Check sheet for the modelled part. Datum: model origin and axes. Units: mm. A direction names the side the tool comes from. Give positions to 0.01 mm unless a question says otherwise; leave off trailing zeros. Order: outer loops, then holes, each group sorted by start corner. A loop starts at its lowest first (then second) coordinate and runs counter-clockwise, first axis right, second up.
Autodesk Inventor part; units mm, degrees
ref_plane "YZ Plane" through (0, 0, 0) normal (1, 0, 0) x (0, 1, 0)
ref_plane "XZ Plane" through (0, 0, 0) normal (0, 1, 0) x (-1, 0, 0)
ref_plane "XY Plane" through (0, 0, 0) normal (0, 0, 1) x (1, 0, 0)
sketch "Sketch2" plane through (0, 0, 0) normal (0, 1, 0) x (-1, 0, 0)
  line L0 (-200, -150) -> (200, -150)
  line L1 (200, -150) -> (200, -200)
  line L2 (-200, -200) -> (-200, -150)
  line L3 (0, -269.3547) -> (0, -73.2831)
  line L4 (200, -200) -> (200, -270)
  line L5 (200, -270) -> (-200, -270)
  line L6 (-200, -270) -> (-200, -200)
  line L7 (200, -150) -> (412.132, 62.132)
  line L8 (200, -150) -> (500, -150) construction
  line L9 (412.132, 62.132) -> (412.132, -57.868)
  line L10 (412.132, -57.868) -> (200, -270)
  line L11 (-200, -150) -> (-412.132, 62.132)
  line L12 (-412.132, 62.132) -> (-412.132, -57.868)
  line L13 (-412.132, -57.868) -> (-200, -270)
  point P0 (0, 0)
  point P1 (0, -175)
  point P2 (412.5, 61.0149)
  dimension "d9" = 400
  dimension "d10" = 50
  dimension "d39" = 70
  dimension "d40" = 200
  dimension "d41" = 45
  dimension "d42" = 120
  dimension "d43" = 150
  dimension "d51" = 300
extrude "Extrusion2" add sketch "Sketch2" along normal blind 150
sketch "Sketch8" plane through (0, 0, 0) normal (0, -1, 0) x (1, 0, 0)
  line L0 (412.132, -57.868) -> (200, -270)
  line L1 (200, -270) -> (-200, -270)
  line L2 (-200, -270) -> (-412.132, -57.868)
  line L3 (-412.132, -57.868) -> (-412.132, 62.132)
  line L4 (-412.132, 62.132) -> (-200, -150)
  line L5 (-200, -150) -> (200, -150)
  line L6 (200, -150) -> (412.132, 62.132)
  line L7 (412.132, 62.132) -> (412.132, -57.868)
  line L8 (-412.132, 62.132) -> (-412.132, 242.132)
  line L9 (412.132, 62.132) -> (412.132, 242.132)
  line L10 (-412.132, 62.132) -> (-412.132, -57.868)
  line L11 (-412.132, -57.868) -> (-200, -270)
  line L12 (-200, -270) -> (200, -270)
  line L13 (200, -270) -> (412.132, -57.868)
  line L14 (412.132, -57.868) -> (412.132, 62.132)
  line L15 (50, 242.132) -> (50, 49.557)
  line L16 (50, 49.557) -> (-50, 49.557)
  line L17 (-50, 49.557) -> (-50, 242.132)
  line L18 (412.132, 242.132) -> (50, 242.132)
  line L19 (-50, 242.132) -> (-412.132, 242.132)
  dimension "d45" = 180
  dimension "d46" = 180
  dimension "d47" = 100
extrude "Extrusion9" add sketch "Sketch8" along normal blind 4
sketch "Sketch9" plane through (0, -4, 0) normal (0, -1, 0) x (1, 0, 0)
  line L0 (200, -270) -> (-200, -270)
  line L1 (-200, -270) -> (-412.132, -57.868)
  line L2 (-412.132, -57.868) -> (-412.132, 242.132)
  line L3 (-412.132, 242.132) -> (-50, 242.132)
  line L4 (-50, 242.132) -> (-50, 49.557)
  line L5 (-50, 49.557) -> (50, 49.557)
  line L6 (50, 49.557) -> (50, 242.132)
  line L7 (50, 242.132) -> (412.132, 242.132)
  line L8 (412.132, 242.132) -> (412.132, -57.868)
  line L9 (412.132, -57.868) -> (200, -270)
  line L10 (200, -270) -> (-200, -270)
  line L11 (-200, -270) -> (-412.132, -57.868)
  line L12 (-412.132, -57.868) -> (-412.132, 242.132)
  line L13 (-412.132, 242.132) -> (-50, 242.132)
  line L14 (-50, 242.132) -> (-50, 49.557)
  line L15 (-50, 49.557) -> (50, 49.557)
  line L16 (50, 49.557) -> (50, 242.132)
  line L17 (50, 242.132) -> (412.132, 242.132)
  line L18 (412.132, 242.132) -> (412.132, -57.868)
  line L19 (412.132, -57.868) -> (200, -270)
  line L20 (200, -270) -> (-200, -270)
  line L21 (-200, -270) -> (-412.132, -57.868)
  line L22 (-412.132, -57.868) -> (-412.132, 242.132)
  line L23 (-412.132, 242.132) -> (-50, 242.132)
  line L24 (-50, 242.132) -> (-50, 49.557)
  line L25 (-50, 49.557) -> (50, 49.557)
  line L26 (50, 49.557) -> (50, 242.132)
  line L27 (50, 242.132) -> (412.132, 242.132)
  line L28 (412.132, 242.132) -> (412.132, -57.868)
  line L29 (412.132, -57.868) -> (200, -270)
  line L30 (250, 110) -> (250, 190)
  line L31 (200, -150) -> (412.132, 62.132)
  line L32 (-200, -150) -> (200, -150)
  line L33 (-412.132, 62.132) -> (-200, -150)
  line L34 (-412.132, 242.132) -> (-412.132, 62.132)
  line L35 (-50, 242.132) -> (-412.132, 242.132)
  line L36 (-50, 49.557) -> (-50, 242.132)
  line L37 (50, 49.557) -> (-50, 49.557)
  line L38 (50, 242.132) -> (50, 49.557)
  line L39 (412.132, 242.132) -> (50, 242.132)
  line L40 (412.132, 62.132) -> (412.132, 242.132)
  line L41 (200, -150) -> (412.132, 62.132)
  line L42 (-200, -150) -> (200, -150)
  line L43 (-412.132, 62.132) -> (-200, -150)
  line L44 (-412.132, 242.132) -> (-412.132, 62.132)
  line L45 (-50, 242.132) -> (-412.132, 242.132)
  line L46 (-50, 49.557) -> (-50, 242.132)
  line L47 (50, 49.557) -> (-50, 49.557)
  line L48 (50, 242.132) -> (50, 49.557)
  line L49 (412.132, 242.132) -> (50, 242.132)
  line L50 (412.132, 62.132) -> (412.132, 242.132)
  circle A0 centre (242.5, 150) radius 2
  circle A1 centre (242.5, 130) radius 2
  line L51 (200, 190) -> (200, 110) construction
  circle A2 centre (157.5, 150) radius 2
  circle A3 centre (157.5, 130) radius 2
  circle A4 centre (42.5, -20.443) radius 2
  circle A5 centre (42.5, -40.443) radius 2
  circle A6 centre (-42.5, -20.443) radius 2
  circle A7 centre (-42.5, -40.443) radius 2
  circle A8 centre (-157.5, 150) radius 2
  circle A9 centre (-157.5, 130) radius 2
  circle A10 centre (-242.5, 150) radius 2
  circle A11 centre (-242.5, 130) radius 2
  point P0 (0, 0)
  point P1 (0, 19.557)
  point P2 (-200, 190)
  dimension "d52" = 4
  dimension "d54" = 7.5
  dimension "d55" = 4
  dimension "d56" = 0
  dimension "d57" = 20
  dimension "d58" = 4
  dimension "d59" = 4
  dimension "d60" = 0
  dimension "d61" = 20
  dimension "d62" = 4
  dimension "d63" = 4
  dimension "d64" = 0
  dimension "d65" = 20
extrude "Extrusion10" cut sketch "Sketch9" against normal up to surface (4 mm away) contours A0 | A1 | A2 | A3 | A4 | A5 | A6 | A7 | A8 | A9 | A10 | A11
properties part number "Charging Dock" material "ABS Plastic"
Q1. Sectioned sample at C-C, the plane z = 40. Record the cut outline in (x, y), plus the area to 3 significant figures.
Q2. Material ranges on line 1 (X direction, y = -2.35, z = 150); line 2 (Z direction, x = -157, y = -2); line 3 (Z direction, x = 42.5, y = -2.5), recorded low to high.
Q3. Sectioned sample at B-B, the plane y = 125.5. Record the cut outline in (x, z), plus the area to 3 significant figures.
Q4. Tool access check on faces 1 (the flat face through (-305, 74, -45)), 2 (the flat face through (-3, 72, -270)). Record the directions out of +Z, -Z, +X, -X, +Y, -Y that give a thin tool (end or side, any length) a straight path to the whole face; none if there is none.
Q5. Sectioned sample at A-A, the plane z = 199. Record the cut outline in (x, y).
Q6. Go/stop test with flat-tipped pins: P1, Ø4.5, axis at x = -157.5, z = 130, coming from the +Y side; P2, Ø4.5, axis at x = 42.5, z = -20.443, coming from the -Y side; P3, Ø6, axis at x = -126, y = 76, coming from the +Z side; P4, Ø2.5, axis at x = 242.5, z = 130, coming from the +Y side (1 decimal). Record where each tip stops, or that it passes through.
Q7. Sectioned sample at D-D, the plane x = 175. Record the cut outline in (y, z).
Filled in:
1. outline: (-412.13, -4) - (412.13, -4) - (412.13, 150) - (390, 150) - (390, 0) - (-390, 0) - (-390, 150) - (-412.13, 150) - close
1. area: 9,940 mm2
2. line 1: x = -412.13 to -244.5, -240.5 to -159.5, -155.5 to -50, 50 to 155.5, 159.5 to 240.5, 244.5 to 412.13
2. line 2: z = -270 to 128.06, 131.94 to 148.06, 151.94 to 242.13
2. line 3: z = -270 to -42.44, -38.44 to -22.44, -18.44 to 49.56
3. outline: (-412.13, -57.87) - (-200, -270) - (200, -270) - (412.13, -57.87) - (412.13, 62.13) - (200, -150) - (-200, -150) - (-412.13, 62.13) - close
3. area: 98,900 mm2
4. face 1: +Z, +Y
4. face 2: -Z, +X, -X, +Y, -Y
5. outline: (-412.13, -4) - (-50, -4) - (-50, 0) - (-412.13, 0) - close; (50, -4) - (412.13, -4) - (412.13, 0) - (50, 0) - close
6. P1: stops at y = 0
6. P2: stops at y = -4
6. P3: stops at z = -150
6. P4: passes through
7. outline: (-4, -270) - (150, -270) - (150, -150) - (0, -150) - (0, 242.13) - (-4, 242.13) - close
